Model file for the job. Use its own axes, mm. Coordinates: 2 decimals unless noted, no trailing zeros. Write each loop counter-clockwise with the first axis right and the second up, starting at its lowest first coordinate (ties: lowest second). Pieces come first, ordered by that corner, then holes. Notation, with made-up numbers: M 62.5,42.5 L 70.5,42.5 A17 ccw 70.5,66.5 Z; hole C 52,48.25 d5. An arc over 180 degrees is marked long. One line per question, with ' | ' between items. Start each with the question number.
(1) Cut at A-A (z = -4). Write the cut outline in (x, y), plus the area to 3 significant figures.
(2) Wall check: probe 1 along X at (y, z) = (-6.5, 37.5). Give the ranges that are in metal, low to high.
(3) Flat gauge pin, fed straight in: pin 1 Ø10 at (x, z) = (75.44, -8.05) entering from -Y (3 decimals). Where does the tip first touch, or does it go through?
(4) Two-plate mould, pull along X, no slides. Class faces 1 (the face through (-125.893, -6.439, -56.875)), 2 (the face through (69.38, -6.44, -9.95)), 3 (the face through (124.369, -6.439, 40.784)): +X half, -X half, draft (parallel to the pull), parting line (faces both ways), or undercut.
from build123d import *

# Parameters (mm, degrees)
F0_W     = 254
F0_H     = 101.6
F1_DEPTH = 12.7
F2_R     = 6.5532
F3_D     = 12.7


with BuildPart() as f1:
    # F0 (on Front) → F1 (new body)
    with BuildSketch(Plane.XZ):
        with Locations((-0.76200068, -8.045138209)):
            Rectangle(F0_W, F0_H)
    extrude(amount=F1_DEPTH)

    # F2
    f2_edges = [f1.edges().sort_by_distance(p)[0] for p in [
        (-127.762001, -6.35, 42.754862),
        (-127.762001, -6.35, -58.845138),
        (126.237999, -6.35, -58.845138),
        (126.237999, -6.35, 42.754862),
    ]]
    fillet(f2_edges, radius=F2_R)

    # F3 (through all)
    with Locations(Plane(origin=(0, 0, 0), x_dir=(1, 0, 0), z_dir=(0, 1, 0))):
        with Locations((-76.96200068, 8.045138209), (75.43799932, 8.045138209)):
            Hole(F3_D / 2)


solid = f1.part
Filled in:
1) outline: M -127.76,-12.7 L -81.86,-12.7 L -81.86,0 L -127.76,0 Z; M -72.07,-12.7 L 70.54,-12.7 L 70.54,0 L -72.07,0 Z; M 80.33,-12.7 L 126.24,-12.7 L 126.24,0 L 80.33,0 Z | area: 2,980 mm²
2) probe 1: -127.63 to 126.11
3) pin 1: through
4) face 1: -X half | face 2: undercut | face 3: +X half
